Geometry check sheet. Reference: the model listing, model coordinates, mm. Coordinates: 2 decimals unless noted, no trailing zeros. Write each loop counter-clockwise with the first axis right and the second up, starting at its lowest first coordinate (ties: lowest second). Pieces come first, ordered by that corner, then holes. Notation, with made-up numbers: (45.5, -33.75) -> (67.5, -33.75) arc R29 cw to (67.5, -1.75) -> close; hole circle Ø7 at (65, 7). An arc over 180 degrees is marked (long way). One line per question, with ' | ' between items.
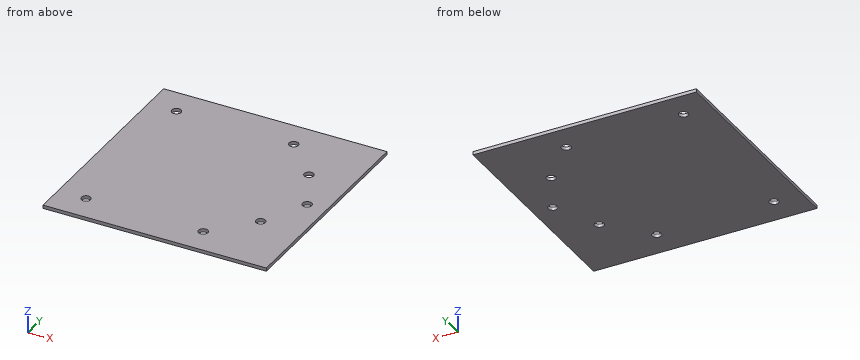
Autodesk Inventor part; units mm, degrees
ref_plane "YZ Plane" through (0, 0, 0) normal (1, 0, 0) x (0, 1, 0)
ref_plane "XZ Plane" through (0, 0, 0) normal (0, 1, 0) x (-1, 0, 0)
ref_plane "XY Plane" through (0, 0, 0) normal (0, 0, 1) x (1, 0, 0)
sketch "Sketch1" plane through (0, 0, 0) normal (0, 0, 1) x (1, 0, 0)
  line L0 (-100, -100) -> (100, -100)
  line L1 (100, -100) -> (100, 100)
  line L2 (100, 100) -> (-100, 100)
  line L3 (-100, 100) -> (-100, -100)
  point P0 (0, 0)
extrude "Extrusion1" add sketch "Sketch1" along normal blind 3
sketch "Sketch2" plane through (0, 0, 3) normal (0, 0, 1) x (1, 0, 0)
  point P0 (0, 0)
  point P1 (-75, 75)
  point P2 (30, 75)
  point P3 (62.5, 40)
  point P4 (82.5001, 0)
  point P5 (62.5, -40)
  point P6 (30, -75)
  point P7 (-75, -75)
hole "Hole1" at (-75, 75, 3) at (30, 75, 3) at (62.5, 40, 3) at (82.5001, 0, 3) at (62.5, -40, 3) at (30, -75, 3) at (-75, -75, 3) direction (0, 0, -1) diameter 8.3 end through all
properties part number "PortaTornillos" material "MDF Medium Density Fiberboard"
1. Cross-section at C-C on y = 75. Record the boundary of the cut face in (x, z), and give its area (3 significant figures).
Worked answers:
outline: (-100, 0) -> (-79.15, 0) -> (-79.15, 3) -> (-100, 3) -> close; (-70.85, 0) -> (25.85, 0) -> (25.85, 3) -> (-70.85, 3) -> close; (34.15, 0) -> (100, 0) -> (100, 3) -> (34.15, 3) -> close | area: 550 mm²
2. Material ranges on line 1 (Y direction, x = 30, z = 0.85); line 2 (X direction, y = -75, z = 1.3); line 3 (Y direction, x = 62.5, z = 1.2), recorded low to high. Write a range as from..to.
Worked answers:
line 1: -100..-79.15, -70.85..70.85, 79.15..100 | line 2: -100..-79.15, -70.85..25.85, 34.15..100 | line 3: -100..-44.15, -35.85..35.85, 44.15..100
3. Go/stop test with a flat-tipped pin: P1, Ø11, axis at x = -75, y = -75, coming from the +Z side. Record where the tip stops, or that it passes through.
Worked answers:
P1: z = 3
4. Cross-section at A-A on y = 0. Record the boundary of the cut face in (x, z).
Worked answers:
outline: (-100, 0) -> (78.35, 0) -> (78.35, 3) -> (-100, 3) -> close; (86.65, 0) -> (100, 0) -> (100, 3) -> (86.65, 3) -> close
5. Cross-section at B-B on x = 30. Record the boundary of the cut face in (y, z).
Worked answers:
outline: (-100, 0) -> (-79.15, 0) -> (-79.15, 3) -> (-100, 3) -> close; (-70.85, 0) -> (70.85, 0) -> (70.85, 3) -> (-70.85, 3) -> close; (79.15, 0) -> (100, 0) -> (100, 3) -> (79.15, 3) -> close
